```python
from build123d import *

# Parameters (mm, degrees)
SKETCH1_W           = 50
SKETCH1_H           = 30
BOSS_EXTRUDE1_DEPTH = 5


with BuildPart() as part:
    # Sketch1 → Boss-Extrude1 (new body)
    with BuildSketch(Plane(origin=(0, 0, 0), x_dir=(1, 0, 0), z_dir=(0, 1, 0))):
        with Locations((25, 15)):
            Rectangle(SKETCH1_W, SKETCH1_H)
        with BuildLine():
            Line((7.5, 27), (42.5, 27))
            ThreePointArc((42.5, 27), (44.5, 25), (42.5, 23))
            Line((42.5, 23), (7.5, 23))
            ThreePointArc((7.5, 23), (5.5, 25), (7.5, 27))
        make_face(mode=Mode.SUBTRACT)
        with BuildLine():
            Line((42.5, 7), (7.5, 7))
            ThreePointArc((7.5, 7), (5.5, 5), (7.5, 3))
            Line((7.5, 3), (42.5, 3))
            ThreePointArc((42.5, 3), (44.5, 5), (42.5, 7))
        make_face(mode=Mode.SUBTRACT)
    extrude(amount=BOSS_EXTRUDE1_DEPTH)


solid = part.part
```
Geometry: final body of the model. Coordinates: model frame, mm. A direction names the side the tool comes from. Round coordinates to 2 decimals unless told otherwise and drop trailing zeros. Loops run counter-clockwise (first coordinate to the right, second up) from the corner with the lowest first, then second, coordinate; pieces in that order, holes last. Notation, with made-up numbers: (21.25, 56.25) -> (29.25, 56.25) arc R6 cw to (29.25, 60.25) -> close; hole circle Ø10 at (-8.5, 48.5). An arc over 180 degrees is marked (long way). Write each question's results on one line, items separated by ' | '.
Item 1: Cut plane A-A on x = 10.5. Return the cut outline in (y, z), and give its area (3 significant figures).
Answers below:
outline: (0, -30) -> (5, -30) -> (5, -27) -> (0, -27) -> close; (0, -23) -> (5, -23) -> (5, -7) -> (0, -7) -> close; (0, -3) -> (5, -3) -> (5, 0) -> (0, 0) -> close | area: 110 mm²
Item 2: Pin query (flat end, axial travel): pin 1 Ø1.5 at (y, z) = (2.5, -9.5) entering from -X. Return the tip coordinate at first contact, or that it passes through.
Answers below:
pin 1: stops at x = 0
Item 3: Cut plane C-C on y = 0.7. Return the cut outline in (x, z).
Answers below:
outline: (0, -30) -> (50, -30) -> (50, 0) -> (0, 0) -> close; hole (7.5, -27) -> (42.5, -27) arc R2 ccw to (42.5, -23) -> (7.5, -23) arc R2 ccw to start; hole (7.5, -7) -> (42.5, -7) arc R2 ccw to (42.5, -3) -> (7.5, -3) arc R2 ccw to start
Item 4: Cut plane B-B on z = -5. Return the cut outline in (x, y), and give its area (3 significant figures).
Answers below:
outline: (0, 0) -> (5.5, 0) -> (5.5, 5) -> (0, 5) -> close; (44.5, 0) -> (50, 0) -> (50, 5) -> (44.5, 5) -> close | area: 55.0 mm²
Item 5: Pull-direction query (Z, two-part tool) for faces 1 (the face through (25, 2, -3)), 2 (the face through (25, 0, -15)), 3 (the face through (25, 2, -30)), 4 (the face through (5.5, 2.5, -5)); classes: pulls with the +Z half, pulls with the -Z half, needs draft (parallel to the pull), parting line crosses it, or undercut.
Answers below:
face 1: undercut | face 2: needs draft | face 3: pulls with the -Z half | face 4: undercut
Item 6: Line query: probe 1 along Z at (x, y) = (32, 4.4); probe 2 along X at (y, z) = (3.95, -23.5). Output: solid intervals per line, ascending. Write a range as [from, to].
Answers below:
probe 1: z = [-30, -27], [-23, -7], [-3, 0] | probe 2: x = [0, 6.18], [43.82, 50]
Item 7: Set-up query: faces 5 (the face through (0, 2, -15)), 6 (the face through (44.5, 2.5, -25)). Return all of +Z, -Z, +X, -X, +Y, -Y with unobstructed straight access to the full face (end or side cutting, diameter ignored); none if empty.
Answers below:
face 5: +Z, -Z, -X, +Y, -Y | face 6: +Y, -Y
